```python
from build123d import *

# Parameters (mm, degrees)
T_LE_DE_BASE_PLI_E1_DEPTH = 56
ENL_V_MAT_EXTRU_1_REACH   = 109.638
ESQUISSE6_R               = 2.5
ESQUISSE6_R_2             = 20
ENL_V_MAT_EXTRU_2_REACH   = 109.638
ESQUISSE7_R               = 2.5


# Sheet-metal steps are written as plain solids
with BuildPart() as part:
    # Esquisse1 → Tôle de base pliée1 (new body)
    with BuildSketch(Plane.XY):
        with BuildLine():
            Line((-65, 0), (-4, 0))
            ThreePointArc((-4, 0), (-1.171572875, -1.171572875), (0, -4))
            Line((0, -4), (0, -65))
            Line((0, -65), (-2, -65))
            Line((-2, -65), (-2, -4))
            ThreePointArc((-2, -4), (-2.585786438, -2.585786438), (-4, -2))
            Line((-4, -2), (-65, -2))
            Line((-65, -2), (-65, 0))
        make_face()
    extrude(amount=T_LE_DE_BASE_PLI_E1_DEPTH)

    # Esquisse6 → Enlèv. mat.-Extru.1 (cut, up to next)
    with BuildSketch(Plane(origin=(0, 0, 0), x_dir=(1, 0, 0), z_dir=(0, 1, 0)), mode=Mode.PRIVATE) as enl_v_mat_extru_1_sk1:
        with Locations(Location((-58, -4.5, 0), (0, 0, 270))):
            Circle(ESQUISSE6_R)
    enl_v_mat_extru_1_tool1 = extrude(enl_v_mat_extru_1_sk1.sketch, amount=-ENL_V_MAT_EXTRU_1_REACH, mode=Mode.PRIVATE) & part.part
    # Esquisse6 → Enlèv. mat.-Extru.1 (cut, up to next)
    with BuildSketch(Plane(origin=(0, 0, 0), x_dir=(1, 0, 0), z_dir=(0, 1, 0)), mode=Mode.PRIVATE) as enl_v_mat_extru_1_sk2:
        with Locations(Location((-11, -4.5, 0), (0, 0, 270))):
            Circle(ESQUISSE6_R)
    enl_v_mat_extru_1_tool2 = extrude(enl_v_mat_extru_1_sk2.sketch, amount=-ENL_V_MAT_EXTRU_1_REACH, mode=Mode.PRIVATE) & part.part
    # Esquisse6 → Enlèv. mat.-Extru.1 (cut, up to next)
    with BuildSketch(Plane(origin=(0, 0, 0), x_dir=(1, 0, 0), z_dir=(0, 1, 0)), mode=Mode.PRIVATE) as enl_v_mat_extru_1_sk3:
        with Locations(Location((-11, -51.5, 0), (0, 0, 270))):
            Circle(ESQUISSE6_R)
    enl_v_mat_extru_1_tool3 = extrude(enl_v_mat_extru_1_sk3.sketch, amount=-ENL_V_MAT_EXTRU_1_REACH, mode=Mode.PRIVATE) & part.part
    # Esquisse6 → Enlèv. mat.-Extru.1 (cut, up to next)
    with BuildSketch(Plane(origin=(0, 0, 0), x_dir=(1, 0, 0), z_dir=(0, 1, 0)), mode=Mode.PRIVATE) as enl_v_mat_extru_1_sk4:
        with Locations(Location((-58, -51.5, 0), (0, 0, 270))):
            Circle(ESQUISSE6_R)
    enl_v_mat_extru_1_tool4 = extrude(enl_v_mat_extru_1_sk4.sketch, amount=-ENL_V_MAT_EXTRU_1_REACH, mode=Mode.PRIVATE) & part.part
    # Esquisse6 → Enlèv. mat.-Extru.1 (cut, up to next)
    with BuildSketch(Plane(origin=(0, 0, 0), x_dir=(1, 0, 0), z_dir=(0, 1, 0)), mode=Mode.PRIVATE) as enl_v_mat_extru_1_sk5:
        with Locations(Location((-34.5, -28, 0), (0, 0, 270))):
            Circle(ESQUISSE6_R_2)
    enl_v_mat_extru_1_tool5 = extrude(enl_v_mat_extru_1_sk5.sketch, amount=-ENL_V_MAT_EXTRU_1_REACH, mode=Mode.PRIVATE) & part.part
    add(enl_v_mat_extru_1_tool1.solids().sort_by_distance((-58, 0, 4.5))[0], mode=Mode.SUBTRACT)
    add(enl_v_mat_extru_1_tool2.solids().sort_by_distance((-11, 0, 4.5))[0], mode=Mode.SUBTRACT)
    add(enl_v_mat_extru_1_tool3.solids().sort_by_distance((-11, 0, 51.5))[0], mode=Mode.SUBTRACT)
    add(enl_v_mat_extru_1_tool4.solids().sort_by_distance((-58, 0, 51.5))[0], mode=Mode.SUBTRACT)
    add(enl_v_mat_extru_1_tool5.solids().sort_by_distance((-34.5, 0, 28))[0], mode=Mode.SUBTRACT)

    # Esquisse7 → Enlèv. mat.-Extru.2 (cut, up to next)
    with BuildSketch(Plane(origin=(0, 0, 0), x_dir=(0, 0, -1), z_dir=(1, 0, 0)), mode=Mode.PRIVATE) as enl_v_mat_extru_2_sk1:
        with Locations(Location((-4.5, -11, 0), (0, 0, 90))):
            Circle(ESQUISSE7_R)
    enl_v_mat_extru_2_tool1 = extrude(enl_v_mat_extru_2_sk1.sketch, amount=-ENL_V_MAT_EXTRU_2_REACH, mode=Mode.PRIVATE) & part.part
    # Esquisse7 → Enlèv. mat.-Extru.2 (cut, up to next)
    with BuildSketch(Plane(origin=(0, 0, 0), x_dir=(0, 0, -1), z_dir=(1, 0, 0)), mode=Mode.PRIVATE) as enl_v_mat_extru_2_sk2:
        with Locations(Location((-4.5, -58, 0), (0, 0, 90))):
            Circle(ESQUISSE7_R)
    enl_v_mat_extru_2_tool2 = extrude(enl_v_mat_extru_2_sk2.sketch, amount=-ENL_V_MAT_EXTRU_2_REACH, mode=Mode.PRIVATE) & part.part
    # Esquisse7 → Enlèv. mat.-Extru.2 (cut, up to next)
    with BuildSketch(Plane(origin=(0, 0, 0), x_dir=(0, 0, -1), z_dir=(1, 0, 0)), mode=Mode.PRIVATE) as enl_v_mat_extru_2_sk3:
        with Locations(Location((-51.5, -58, 0), (0, 0, 90))):
            Circle(ESQUISSE7_R)
    enl_v_mat_extru_2_tool3 = extrude(enl_v_mat_extru_2_sk3.sketch, amount=-ENL_V_MAT_EXTRU_2_REACH, mode=Mode.PRIVATE) & part.part
    # Esquisse7 → Enlèv. mat.-Extru.2 (cut, up to next)
    with BuildSketch(Plane(origin=(0, 0, 0), x_dir=(0, 0, -1), z_dir=(1, 0, 0)), mode=Mode.PRIVATE) as enl_v_mat_extru_2_sk4:
        with Locations(Location((-51.5, -11, 0), (0, 0, 90))):
            Circle(ESQUISSE7_R)
    enl_v_mat_extru_2_tool4 = extrude(enl_v_mat_extru_2_sk4.sketch, amount=-ENL_V_MAT_EXTRU_2_REACH, mode=Mode.PRIVATE) & part.part
    add(enl_v_mat_extru_2_tool1.solids().sort_by_distance((0, -11, 4.5))[0], mode=Mode.SUBTRACT)
    add(enl_v_mat_extru_2_tool2.solids().sort_by_distance((0, -58, 4.5))[0], mode=Mode.SUBTRACT)
    add(enl_v_mat_extru_2_tool3.solids().sort_by_distance((0, -58, 51.5))[0], mode=Mode.SUBTRACT)
    add(enl_v_mat_extru_2_tool4.solids().sort_by_distance((0, -11, 51.5))[0], mode=Mode.SUBTRACT)


solid = part.part
```
Geometry check sheet. Reference: the model listing, model coordinates, mm. A direction names the side the tool comes from. Coordinates: 2 decimals unless noted, no trailing zeros. Loops run counter-clockwise (first coordinate to the right, second up) from the corner with the lowest first, then second, coordinate; pieces in that order, holes last.
Item 1: Release check for a two-part mould opening along Y. For faces 1 (the face through (-11.96, -0.99, 53.81)), 2 (the face through (-1, -13.5, 4.6)), 3 (the face through (-1, -65, 28)), 4 (the face through (-42, 0, 9)) record: released by +Y, released by -Y, zero draft, split by the parting line, or undercut.
Item 2: Sectioned sample at D-D, the plane y = -11. Record the boundary of the cut face in (x, z), then the cut area to 3 significant figures.
Item 3: Sectioned sample at C-C, the plane x = -56.5. Record the boundary of the cut face in (y, z), then the cut area to 3 significant figures.
Item 4: Sectioned sample at B-B, the plane z = 28. Record the boundary of the cut face in (x, y), then the cut area to 3 significant figures.
Item 5: Go/stop test with flat-tipped pins: pin 1 Ø5 at (y, z) = (-23, 47) entering from -X; pin 2 Ø4.5 at (x, z) = (-11, 4.5) entering from +Y; pin 3 Ø6 at (x, z) = (-58, 4.5) entering from -Y. Record where each tip stops, or that it passes through.
Item 6: Access from +Z, -Z, +X, -X, +Y, -Y to the whole of each face (thin tool, end or side, straight path). Record for faces 5 (the face through (-2, -35, 28)), 6 (the face through (-13, -1, 6)).
Item 7: Thickness scan on line 1 (Z direction, x = -0.9, y = -58); line 2 (Y direction, x = -1, z = 51); line 3 (X direction, y = -0.8, z = 51.5). Record the ranges inside material, lowest first.
Item 8: Sectioned sample at A-A, the plane x = -34.5. Record the boundary of the cut face in (y, z), then the cut area to 3 significant figures.
Check result:
1. face 1: zero draft
1. face 2: undercut
1. face 3: released by -Y
1. face 4: released by +Y
2. outline: (-2, 0) - (0, 0) - (0, 2) - (-2, 2) - close; (-2, 7) - (0, 7) - (0, 49) - (-2, 49) - close; (-2, 54) - (0, 54) - (0, 56) - (-2, 56) - close
2. area: 92.0 mm2
3. outline: (-2, 0) - (0, 0) - (0, 2.5) - (-2, 2.5) - close; (-2, 6.5) - (0, 6.5) - (0, 49.5) - (-2, 49.5) - close; (-2, 53.5) - (0, 53.5) - (0, 56) - (-2, 56) - close
3. area: 96.0 mm2
4. outline: (-65, -2) - (-54.5, -2) - (-54.5, 0) - (-65, 0) - close; (-14.5, -2) - (-4, -2) arc R2 cw to (-2, -4) - (-2, -65) - (0, -65) - (0, -4) arc R4 ccw to (-4, 0) - (-14.5, 0) - close
4. area: 173 mm2
5. pin 1: stops at x = -2
5. pin 2: passes through
5. pin 3: stops at y = -2
6. face 5: +Z, -Z, -X, -Y
6. face 6: +Y, -Y
7. line 1: z = 0 to 2, 7 to 49, 54 to 56
7. line 2: y = -65 to -60.45, -55.55 to -13.45, -8.55 to -1.35
7. line 3: x = -65 to -60.5, -55.5 to -13.5, -8.5 to -1.6
8. outline: (-2, 0) - (0, 0) - (0, 8) - (-2, 8) - close; (-2, 48) - (0, 48) - (0, 56) - (-2, 56) - close
8. area: 32.0 mm2
